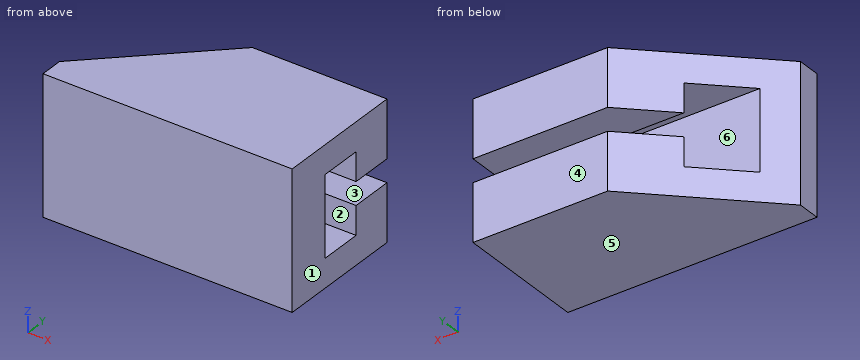
```python
from build123d import *

# Parameters (mm, degrees)
SKETCH1_W               = 87
SKETCH1_H               = 48
BOSS_EXTRUDE1_DEPTH     = 46
CUT_EXTRUDE1_DEPTH      = 68.707089732
CUT_EXTRUDE1_DEPTH_BACK = 68.707089732
CUT_EXTRUDE2_DEPTH      = 68.707089732
CUT_EXTRUDE2_DEPTH_BACK = 68.707089732


with BuildPart() as part:
    # Sketch1 → Boss-Extrude1 (new body)
    with BuildSketch(Plane(origin=(0, 0, 0), x_dir=(1, 0, 0), z_dir=(0, 1, 0))):
        Rectangle(SKETCH1_W, SKETCH1_H)
    extrude(amount=BOSS_EXTRUDE1_DEPTH)

    # Sketch2 → Cut-Extrude1 (cut, two sides: drawn at the far end of the back side and taken through both)
    with BuildSketch(Plane(origin=(0, 0, 0), x_dir=(0, 0, -1), z_dir=(1, 0, 0)).offset(-CUT_EXTRUDE1_DEPTH_BACK)):
        Polygon((4, 31), (14, 31), (14, 16), (-14, 16), (-14, 31), (-4, 31), (-4, 46), (4, 46), align=None)
    extrude(amount=CUT_EXTRUDE1_DEPTH + CUT_EXTRUDE1_DEPTH_BACK, mode=Mode.SUBTRACT)

    # Sketch3 → Cut-Extrude2 (cut, two sides: drawn at the far end of the back side and taken through both)
    with BuildSketch(Plane.XY.offset(-CUT_EXTRUDE2_DEPTH_BACK)):
        Polygon((-43.5, 46), (-43.5, 8), (-3.5, 46), align=None)
    extrude(amount=CUT_EXTRUDE2_DEPTH + CUT_EXTRUDE2_DEPTH_BACK, mode=Mode.SUBTRACT)


solid = part.part
```
Check sheet for the modelled part. Datum: model origin and axes. Units: mm. Face numbers are marked on the shaded views. A direction names the side the tool comes from. Give positions to 0.01 mm unless a question says otherwise; leave off trailing zeros. Write each loop counter-clockwise with the first axis right and the second up, starting at its lowest first coordinate (ties: lowest second). Pieces come first, ordered by that corner, then holes. Notation, with made-up numbers: (-34.75, 39) - (22.25, 39) arc R33 ccw to (22.25, 77) - close; hole circle Ø2 at (-7.75, 20). An arc over 180 degrees is marked (long way). Answer as a JSON object with one key per item and string values. Group by question number.
1) Release check for a two-part mould opening along Y. For the marked faces 4, 5 and 6 record: pulls with the +Y half, pulls with the -Y half, needs draft (parallel to the pull), parting line crosses it, or undercut.
2) Sectioned sample at D-D (z = -2). Record the cut outline in (x, y), then the cut area to 3 significant figures.
3) Thickness scan on probe 1 along Z at (x, y) = (35.5, 32); probe 2 along Z at (x, y) = (38, 21); probe 3 along Y at (x, z) = (17.5, 5). Record the ranges inside material, lowest first. Write a range as from..to.
4) Sectioned sample at B-B (y = 35.5). Record the cut outline in (x, z), then the cut area to 3 significant figures.
5) Sectioned sample at A-A (z = 5.5). Record the cut outline in (x, y).
6) Sectioned sample at C-C (x = -16.5). Record the cut outline in (y, z).
7) Access from +Z, -Z, +X, -X, +Y, -Y to the whole of each face (thin tool, end or side, straight path). Record for the marked faces 1, 2 and 3.
Geometry results:
{
 "1": {"face 4": "pulls with the +Y half", "face 5": "needs draft", "face 6": "undercut"},
 "2": {"outline": "(-43.5, 0) - (43.5, 0) - (43.5, 16) - (-35.08, 16) - (-43.5, 8) - close", "area": "1,360 mm^2"},
 "3": {"probe 1": "z = -24..-4, 4..24", "probe 2": "z = -24..-14, 14..24", "probe 3": "y = 0..16, 31..46"},
 "4": {"outline": "(-14.55, -24) - (43.5, -24) - (43.5, -4) - (-14.55, -4) - close; (-14.55, 4) - (43.5, 4) - (43.5, 24) - (-14.55, 24) - close", "area": "2,320 mm^2"},
 "5": {"outline": "(-43.5, 0) - (43.5, 0) - (43.5, 16) - (-35.08, 16) - (-43.5, 8) - close; (-19.29, 31) - (43.5, 31) - (43.5, 46) - (-3.5, 46) - close"},
 "6": {"outline": "(0, -24) - (33.65, -24) - (33.65, -4) - (31, -4) - (31, -14) - (16, -14) - (16, 14) - (31, 14) - (31, 4) - (33.65, 4) - (33.65, 24) - (0, 24) - close"},
 "7": {"face 1": "+Z, -Z, +X, +Y, -Y", "face 2": "+X, -X", "face 3": "+X, -X, +Y"}
}
